For this review, take the finished solid that the model builds, in its own axes (mm). A direction names the side the tool comes from. Give positions to 0.01 mm unless a question says otherwise; leave off trailing zeros. Write each loop counter-clockwise with the first axis right and the second up, starting at its lowest first coordinate (ties: lowest second). Pieces come first, ordered by that corner, then holes. Notation, with made-up numbers: M 86.5,-16.5 L 126.5,-16.5 A15 cw 126.5,11.5 Z; hole C 4.25,86 d7. An arc over 180 degrees is marked long. Use one line per item in the form item = value. Start each with the question number.
Q1. Consider section A-A on z = 15. Write out the cut boundary in (x, y), and give its area (3 significant figures).
Q2. Mouldability with a two-part tool opening along Z and no side actions: class faces 1 (the cylindrical face through (62.56, 2.03, 14.37)), 2 (the flat face through (46.766, 46.37, 9.529)), 3 (the flat face through (-59.1, 37.985, 1.071)) as released by +Z, released by -Z, zero draft, split by the parting line, or undercut.
Q3. Consider section C-C on x = 0. Write out the cut boundary in (y, z), and give its area (3 significant figures).
Q4. Consider section B-B on y = 17. Write out the cut boundary in (x, z).
Q5. Consider section D-D on x = 18. Write out the cut boundary in (y, z).
Q6. For probe 1 along Y at (x, z) = (-1, 3.25); probe 2 along X at (y, z) = (13, 4); probe 3 along X at (y, z) = (14.5, 9), list the stretches that pass through material, from the lowest coordinate up. Write a range as [from, to].
Q7. Clearance check with flat-ended pins moving along their axes: pin 1 Ø6 at (x, z) = (-33.5, 5) entering from +Y; pin 2 Ø8 at (x, z) = (5, 11) entering from -Y; pin 3 Ø9 at (x, z) = (-63.5, 9) entering from +Y; pin 4 Ø2.5 at (x, z) = (-64.08, 15) entering from -Y. State where each tip first meets the part, or that it passes through.
Q8. Tool access review of faces 4 (the flat face through (54.91, 34.62, 6.06)), 5 (the flat face through (36.1, 50.24, 7.92)), 6 (the flat face through (60.87, 32.586, 5.446)): name each direction out of +Z, -Z, +X, -X, +Y, -Y from which nothing blocks a thin tool from reaching the whole face with its end or side.
```python
from build123d import *

# Parameters (mm, degrees)
EXTRUDE_1_DEPTH     = 20
EXTRUDE_2_DEPTH     = 20
CUT_EXTRUDE_1_REACH = 99.146
CUT_EXTRUDE_2_REACH = 99.146
EXTRUDE_3_DEPTH     = 4
EXTRUDE_4_DEPTH     = 4
CUT_EXTRUDE_3_REACH = 113.665
SKETCH_8_R          = 1.65
FILLET_1_R          = 2
CUT_EXTRUDE_4_REACH = 113.513
SKETCH_9_R          = 1.65
SKETCH_10_W         = 10
SKETCH_10_H         = 20
EXTRUDE_5_DEPTH     = 4
CUT_EXTRUDE_5_REACH = 94.836
SKETCH_11_R         = 1.65


with BuildPart() as part:
    # ｽｹｯﾁ1 → ﾎﾞｽ - 押し出し1 (new body)
    with BuildSketch(Plane.XY):
        with BuildLine():
            Line((-57.15, 0), (-60.15, 0))
            ThreePointArc((-60.15, 0), (0, 60.15), (60.15, 0))
            Line((60.15, 0), (57.15, 0))
            ThreePointArc((57.15, 0), (0, 57.15), (-57.15, 0))
        make_face()
    extrude(amount=EXTRUDE_1_DEPTH)

    # ｽｹｯﾁ3 → ﾎﾞｽ - 押し出し2 (add)
    with BuildSketch(Plane.XY.offset(20)):
        Polygon((-41.94056807, 41.94056807), (-34.869500258, 49.011635881), (-43.708335023, 57.850470646), (-57.850470646, 43.708335023), (-49.011635881, 34.869500258), align=None)
        Polygon((57.850470646, 43.708335023), (49.011635881, 34.869500258), (41.94056807, 41.94056807), (34.869500258, 49.011635881), (43.708335023, 57.850470646), align=None)
    extrude(amount=-EXTRUDE_2_DEPTH)

    # ｽｹｯﾁ4 → ｶｯﾄ - 押し出し1 (cut, up to next)
    with BuildSketch(Plane(origin=(-7.071067812, -7.071067812, 0), x_dir=(0, 0, 1), z_dir=(-0.7071067811865431, -0.7071067811865519, 0)), mode=Mode.PRIVATE) as cut_extrude_1_sk1:
        Polygon((0, 71.812920178), (20, 59.312920178), (20, 71.812920178), align=None)
    cut_extrude_1_tool1 = extrude(cut_extrude_1_sk1.sketch, amount=-CUT_EXTRUDE_1_REACH, mode=Mode.PRIVATE) & part.part
    add(cut_extrude_1_tool1.solids().sort_by_distance((-54.904192, 40.762057, 13.333333))[0], mode=Mode.SUBTRACT)

    # ｽｹｯﾁ5 → ｶｯﾄ - 押し出し2 (cut, up to next)
    with BuildSketch(Plane(origin=(7.071067812, -7.071067812, 0), x_dir=(0, 0, -1), z_dir=(0.7071067811865431, -0.7071067811865519, 0)), mode=Mode.PRIVATE) as cut_extrude_2_sk1:
        Polygon((0, 71.812920178), (-20, 59.312920178), (-20, 71.812920178), align=None)
    cut_extrude_2_tool1 = extrude(cut_extrude_2_sk1.sketch, amount=-CUT_EXTRUDE_2_REACH, mode=Mode.PRIVATE) & part.part
    add(cut_extrude_2_tool1.solids().sort_by_distance((54.904192, 40.762057, 13.333333))[0], mode=Mode.SUBTRACT)

    # ｽｹｯﾁ6 → ﾎﾞｽ - 押し出し3 (add)
    with BuildSketch(Plane(origin=(-36.515525634, 36.515525634, 32.275469743), x_dir=(0.7991544988642271, 0.4135236263174359, 0.4362915280203637), z_dir=(-0.5996253511966934, 0.5996253511966858, 0.5299989400031792))):
        Polygon((-26.82708742, 25.275306051), (-35.402016678, 20.130348497), (-30.257059123, 11.55541924), (-21.682129866, 16.700376794), align=None)
        Polygon((4.042657905, 32.135249457), (-4.532271352, 26.990291903), (-9.677228906, 35.56522116), (-1.102299649, 40.710178714), align=None)
    extrude(amount=-EXTRUDE_3_DEPTH)

    # ｽｹｯﾁ7 → ﾎﾞｽ - 押し出し4 (add)
    with BuildSketch(Plane(origin=(36.515525634, 36.515525634, 32.275469743), x_dir=(0.7991544988642272, -0.41352362631743567, -0.43629152802036364), z_dir=(0.5996253511966931, 0.5996253511966856, 0.5299989400031795))):
        Polygon((9.677228906, 35.56522116), (4.532271352, 26.990291903), (-4.042657905, 32.135249457), (1.102299649, 40.710178714), align=None)
        Polygon((30.257059123, 11.55541924), (35.402016678, 20.130348497), (26.82708742, 25.275306051), (21.682129866, 16.700376794), align=None)
    extrude(amount=-EXTRUDE_4_DEPTH)

    # ｽｹｯﾁ8 → ｶｯﾄ - 押し出し3 (cut, up to next)
    with BuildSketch(Plane(origin=(36.515525634, 36.515525634, 32.275469743), x_dir=(0.7991544988642272, -0.41352362631743567, -0.43629152802036364), z_dir=(0.5996253511966931, 0.5996253511966856, 0.5299989400031795)), mode=Mode.PRIVATE) as cut_extrude_3_sk1:
        with Locations(Location((2.817285501, 33.850235308, 0), (0, 0, 149.036243468))):
            Circle(SKETCH_8_R)
    cut_extrude_3_tool1 = extrude(cut_extrude_3_sk1.sketch, amount=-CUT_EXTRUDE_3_REACH, mode=Mode.PRIVATE) & part.part
    # ｽｹｯﾁ8 → ｶｯﾄ - 押し出し3 (cut, up to next)
    with BuildSketch(Plane(origin=(36.515525634, 36.515525634, 32.275469743), x_dir=(0.7991544988642272, -0.41352362631743567, -0.43629152802036364), z_dir=(0.5996253511966931, 0.5996253511966856, 0.5299989400031795)), mode=Mode.PRIVATE) as cut_extrude_3_sk2:
        with Locations(Location((28.542073272, 18.415362646, 0), (0, 0, 149.036243468))):
            Circle(SKETCH_8_R)
    cut_extrude_3_tool2 = extrude(cut_extrude_3_sk2.sketch, amount=-CUT_EXTRUDE_3_REACH, mode=Mode.PRIVATE) & part.part
    add(cut_extrude_3_tool1.solids().sort_by_distance((37.33022, 58.543423, 6.432027))[0], mode=Mode.SUBTRACT)
    add(cut_extrude_3_tool2.solids().sort_by_distance((58.543423, 37.33022, 6.432027))[0], mode=Mode.SUBTRACT)

    # ﾌｨﾚｯﾄ1
    fillet_1_edges = [part.edges().sort_by_distance(p)[0] for p in [
        (50.779402834, 50.779402834, 0),
        (-50.779402834, 50.779402834, 0),
    ]]
    fillet(fillet_1_edges, radius=FILLET_1_R)

    # ｽｹｯﾁ9 → ｶｯﾄ - 押し出し4 (cut, up to next)
    with BuildSketch(Plane(origin=(-36.515525634, 36.515525634, 32.275469743), x_dir=(0.7991544988642271, 0.4135236263174359, 0.4362915280203637), z_dir=(-0.5996253511966934, 0.5996253511966858, 0.5299989400031792)), mode=Mode.PRIVATE) as cut_extrude_4_sk1:
        with Locations(Location((-2.817285501, 33.850235308, 0), (0, 0, 210.963756532))):
            Circle(SKETCH_9_R)
    cut_extrude_4_tool1 = extrude(cut_extrude_4_sk1.sketch, amount=-CUT_EXTRUDE_4_REACH, mode=Mode.PRIVATE) & part.part
    # ｽｹｯﾁ9 → ｶｯﾄ - 押し出し4 (cut, up to next)
    with BuildSketch(Plane(origin=(-36.515525634, 36.515525634, 32.275469743), x_dir=(0.7991544988642271, 0.4135236263174359, 0.4362915280203637), z_dir=(-0.5996253511966934, 0.5996253511966858, 0.5299989400031792)), mode=Mode.PRIVATE) as cut_extrude_4_sk2:
        with Locations(Location((-28.542073272, 18.415362646, 0), (0, 0, 210.963756532))):
            Circle(SKETCH_9_R)
    cut_extrude_4_tool2 = extrude(cut_extrude_4_sk2.sketch, amount=-CUT_EXTRUDE_4_REACH, mode=Mode.PRIVATE) & part.part
    add(cut_extrude_4_tool1.solids().sort_by_distance((-37.33022, 58.543423, 6.432027))[0], mode=Mode.SUBTRACT)
    add(cut_extrude_4_tool2.solids().sort_by_distance((-58.543423, 37.33022, 6.432027))[0], mode=Mode.SUBTRACT)

    # ｽｹｯﾁ10 → ﾎﾞｽ - 押し出し5 (add)
    with BuildSketch(Plane.XZ):
        with Locations((-63.15, 10)):
            Rectangle(SKETCH_10_W, SKETCH_10_H)
        with Locations((63.15, 10)):
            Rectangle(SKETCH_10_W, SKETCH_10_H)
    extrude(amount=-EXTRUDE_5_DEPTH)

    # ｽｹｯﾁ11 → ｶｯﾄ - 押し出し5 (cut, up to next)
    with BuildSketch(Plane(origin=(0, 4, 0), x_dir=(1, 0, 0), z_dir=(0, 1, 0)), mode=Mode.PRIVATE) as cut_extrude_5_sk1:
        with Locations(Location((64.0834259, -5, 0), (0, 0, 180))):
            Circle(SKETCH_11_R)
    cut_extrude_5_tool1 = extrude(cut_extrude_5_sk1.sketch, amount=-CUT_EXTRUDE_5_REACH, mode=Mode.PRIVATE) & part.part
    # ｽｹｯﾁ11 → ｶｯﾄ - 押し出し5 (cut, up to next)
    with BuildSketch(Plane(origin=(0, 4, 0), x_dir=(1, 0, 0), z_dir=(0, 1, 0)), mode=Mode.PRIVATE) as cut_extrude_5_sk2:
        with Locations(Location((64.0834259, -15, 0), (0, 0, 180))):
            Circle(SKETCH_11_R)
    cut_extrude_5_tool2 = extrude(cut_extrude_5_sk2.sketch, amount=-CUT_EXTRUDE_5_REACH, mode=Mode.PRIVATE) & part.part
    # ｽｹｯﾁ11 → ｶｯﾄ - 押し出し5 (cut, up to next)
    with BuildSketch(Plane(origin=(0, 4, 0), x_dir=(1, 0, 0), z_dir=(0, 1, 0)), mode=Mode.PRIVATE) as cut_extrude_5_sk3:
        with Locations(Location((-64.0834259, -15, 0), (0, 0, 180))):
            Circle(SKETCH_11_R)
    cut_extrude_5_tool3 = extrude(cut_extrude_5_sk3.sketch, amount=-CUT_EXTRUDE_5_REACH, mode=Mode.PRIVATE) & part.part
    # ｽｹｯﾁ11 → ｶｯﾄ - 押し出し5 (cut, up to next)
    with BuildSketch(Plane(origin=(0, 4, 0), x_dir=(1, 0, 0), z_dir=(0, 1, 0)), mode=Mode.PRIVATE) as cut_extrude_5_sk4:
        with Locations(Location((-64.0834259, -5, 0), (0, 0, 180))):
            Circle(SKETCH_11_R)
    cut_extrude_5_tool4 = extrude(cut_extrude_5_sk4.sketch, amount=-CUT_EXTRUDE_5_REACH, mode=Mode.PRIVATE) & part.part
    add(cut_extrude_5_tool1.solids().sort_by_distance((64.083426, 4, 5))[0], mode=Mode.SUBTRACT)
    add(cut_extrude_5_tool2.solids().sort_by_distance((64.083426, 4, 15))[0], mode=Mode.SUBTRACT)
    add(cut_extrude_5_tool3.solids().sort_by_distance((-64.083426, 4, 15))[0], mode=Mode.SUBTRACT)
    add(cut_extrude_5_tool4.solids().sort_by_distance((-64.083426, 4, 5))[0], mode=Mode.SUBTRACT)


solid = part.part
```
Working result:
q1.outline = M -68.15,0 L -65.73,0 L -65.73,4 L -68.15,4 Z; M -62.43,0 L -57.15,0 A57.15 cw 57.15,0 L 62.43,0 L 62.43,4 L 60.02,4 A60.15 ccw 49.01,34.87 L 51.22,37.08 L 37.08,51.22 L 34.87,49.01 A60.15 ccw -34.87,49.01 L -37.08,51.22 L -51.22,37.08 L -49.01,34.87 A60.15 ccw -60.02,4 L -62.43,4 Z; M 65.73,0 L 68.15,0 L 68.15,4 L 65.73,4 Z
q1.area = 693 mm²
q2.face_1 = undercut
q2.face_2 = released by +Z
q2.face_3 = released by -Z
q3.outline = M 57.15,0 L 60.15,0 L 60.15,20 L 57.15,20 Z
q3.area = 60.0 mm²
q4.outline = M -57.7,0 L -54.56,0 L -54.56,20 L -57.7,20 Z; M 54.56,0 L 57.7,0 L 57.7,20 L 54.56,20 Z
q5.outline = M 54.24,0 L 57.39,0 L 57.39,20 L 54.24,20 Z
q6.probe_1 = [57.14, 60.14]
q6.probe_2 = [-58.73, -55.65], [55.65, 58.73]
q6.probe_3 = [-58.38, -55.28], [55.28, 58.38]
q7.pin_1 = 63.7
q7.pin_2 = 56.44
q7.pin_3 = 36.11
q7.pin_4 = through
q8.face_4 = -Z
q8.face_5 = none
q8.face_6 = +Z, -Z, +X
